Answer from the drawing. Dimensions are ordinates in mm from the lowest x, y and z of the part. A direction names the side the tool comes from. Give positions to 0.01 mm unless a question says otherwise; leave off trailing zeros. Write each loop counter-clockwise with the first axis right and the second up, starting at its lowest first coordinate (ties: lowest second). Pieces come first, ordered by that corner, then holes.
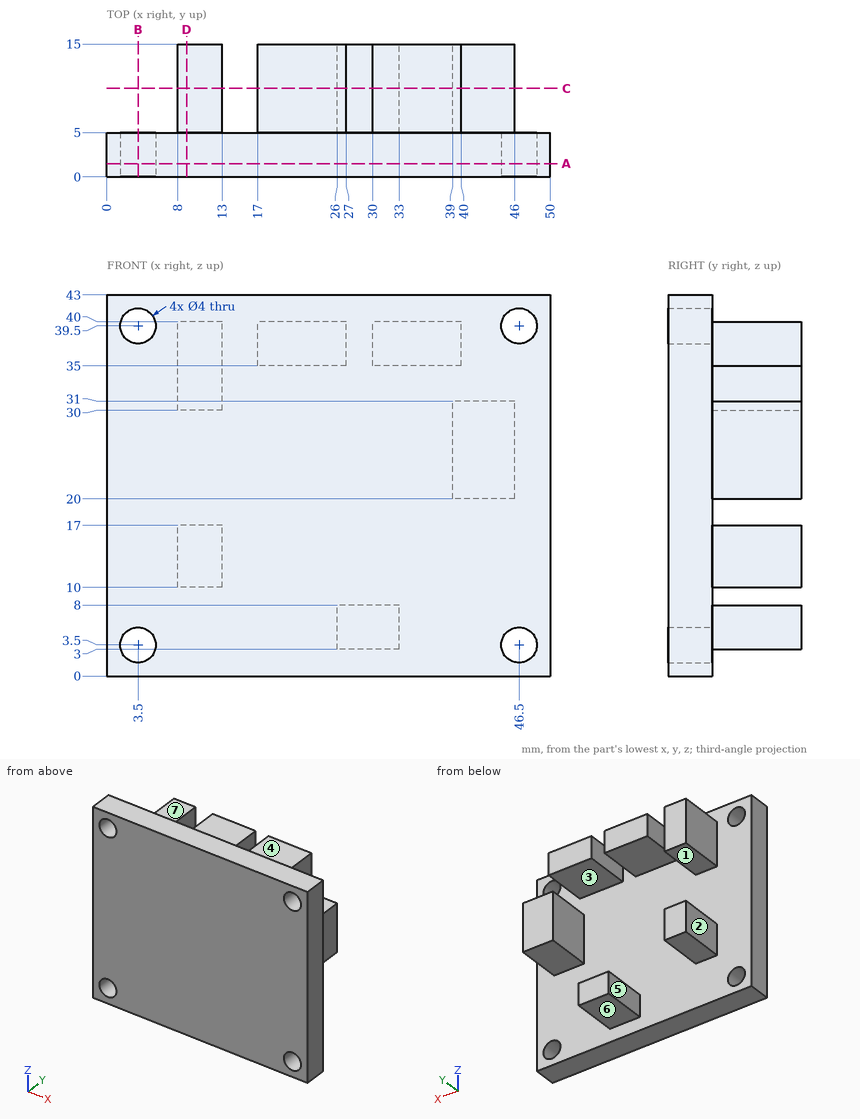
Item 1: A cutting plane is placed at B-B, the plane x = 3.5. Give the vertices of the cut face in (y, z).
Conclusion:
outline: (0, 0) - (5, 0) - (5, 1.5) - (0, 1.5) - close; (0, 5.5) - (5, 5.5) - (5, 37.5) - (0, 37.5) - close; (0, 41.5) - (5, 41.5) - (5, 43) - (0, 43) - close
Item 2: Each of these flat-tipped pins is pushed along its axis until it touches: P1, Ø1.5, axis at x = 11, y = 12, coming from the +Z side; P2, Ø5, axis at x = 28, y = 6.5, coming from the +Z side; P3, Ø5.5, axis at x = 10.5, y = 11.5, coming from the -Z side; P4, Ø8, axis at y = 12, z = 27, coming from the +X side. Where does it stop, or does it pass through?
Conclusion:
P1: stops at z = 40
P2: stops at z = 43
P3: stops at z = 10
P4: stops at x = 46
Item 3: Which of the six approach directions +Z, -Z, +X, -X, +Y, -Y give full straight-line access (tool end or side, diameter ignored) to the marked faces 5, 6 and 7?
Conclusion:
face 5: -Z, -X, +Y
face 6: -Z, +X, -X, +Y
face 7: +Z, +X, -X, +Y
Item 4: Determine the mould class of the marked faces 1, 2, 3 and 4 for opening direction Z: pulls with the +Z half, pulls with the -Z half, needs draft (parallel to the pull), parting line crosses it, or undercut.
Conclusion:
face 1: undercut
face 2: needs draft
face 3: undercut
face 4: pulls with the +Z half
Item 5: A cutting plane is placed at C-C, the plane y = 10. Give the vertices of the cut face in (x, z).
Conclusion:
outline: (8, 10) - (13, 10) - (13, 17) - (8, 17) - close; (8, 30) - (13, 30) - (13, 40) - (8, 40) - close; (17, 35) - (27, 35) - (27, 40) - (17, 40) - close; (26, 3) - (33, 3) - (33, 8) - (26, 8) - close; (30, 35) - (40, 35) - (40, 40) - (30, 40) - close; (39, 20) - (46, 20) - (46, 31) - (39, 31) - close
Item 6: Consider probe 1 along X at (y, z) = (12.75, 38); probe 2 along X at (y, z) = (2.05, 3.5); probe 3 along Z at (x, y) = (32, 6.75). Determine where each line is inside the solid, lowest interval first.
Conclusion:
probe 1: x = 8 to 13, 17 to 27, 30 to 40
probe 2: x = 0 to 1.5, 5.5 to 44.5, 48.5 to 50
probe 3: z = 3 to 8, 35 to 40
Item 7: A cutting plane is placed at D-D, the plane x = 9. Give the vertices of the cut face in (y, z).
Conclusion:
outline: (0, 0) - (5, 0) - (5, 10) - (15, 10) - (15, 17) - (5, 17) - (5, 30) - (15, 30) - (15, 40) - (5, 40) - (5, 43) - (0, 43) - close
Item 8: A cutting plane is placed at A-A, the plane y = 1.5. Give the vertices of the cut face in (x, z), plus the area to 3 significant figures.
Conclusion:
outline: (0, 0) - (50, 0) - (50, 43) - (0, 43) - close; hole circle Ø4 at (3.5, 3.5); hole circle Ø4 at (3.5, 39.5); hole circle Ø4 at (46.5, 3.5); hole circle Ø4 at (46.5, 39.5)
area: 2,100 mm2
